Could you check a few things on this model? Use its own coordinates, in mm. A direction names the side the tool comes from. Round coordinates to 2 decimals unless told otherwise and drop trailing zeros. Loops run counter-clockwise (first coordinate to the right, second up) from the corner with the lowest first, then second, coordinate; pieces in that order, holes last. Notation, with made-up numbers: (86, 10) -> (100, 10) arc R23 ccw to (100, 20) -> close; hole circle Ø11 at (-4, 70). An arc over 180 degrees is marked (long way). Write each question's results on one line, items separated by ' | '. Start each with the question number.
1) Imagine slicing it at B-B, the plane x = -4. List the corners of the cut face in (y, z) for me, plus the area to 3 significant figures.
2) For P1, Ø2, axis at x = -17, y = 1, coming from the +Z side; P2, Ø3, axis at x = 12, y = 2.5, coming from the -Z side; P3, Ø0.9, axis at x = -1, z = 1.5, coming from the +Y side, each with a flat end and sliding along its axis, tell me the tip position at first contact or that it passes through.
3) If I drill on probe 1 along X at (y, z) = (0.8, 0); probe 2 along X at (y, z) = (0.5, 9.5); probe 3 along X at (y, z) = (1.5, 0), over which ranges is the centre line in solid material (lowest first)?
4) We'd pull the mould along Z, two halves only. Please class faces 3 (the cylindrical face through (0.07, 0.99, 10.6)), 4 (the flat face through (0.14, 3.521, -12.246)), 5 (the cylindrical face through (-22.497, 0.986, -0.275)): pulls with the +Z half, pulls with the -Z half, needs draft (parallel to the pull), parting line crosses it, or undercut.
5) Imagine slicing it at A-A, the plane z = 0. List the corners of the cut face in (x, y) for me, plus the area to 3 significant figures.
6) Which directions (+Z, -Z, +X, -X, +Y, -Y) give clear straight access to the entire face, cutting with the end or side of a thin tool? Please do faces 1 (the cylindrical face through (-19.27, 1.01, 1.22)), 2 (the flat face through (1, 2, -7)).
from build123d import *
from OCP.BRepFilletAPI import BRepFilletAPI_MakeChamfer

# Parameters (mm, degrees)
BOSS_EXTRUDE1_DEPTH = 2
SKETCH2_R           = 9.349999999999996
CUT_EXTRUDE1_DEPTH  = 26.81666128685116
BOSS_EXTRUDE2_DEPTH = 3
CHAMFER1_SIZE       = 3
CHAMFER1_SIZE2      = 0.5
SKETCH4_W           = 15.000000000000002
SKETCH4_H           = 12
CUT_EXTRUDE2_DEPTH  = 1
CHAMFER2_SIZE       = 1
CHAMFER2_SIZE_2     = 2
SKETCH5_R           = 1.6000000000000005
SKETCH5_R_2         = 0.75
SKETCH5_R_3         = 0.7500000000000004
CUT_EXTRUDE3_DEPTH  = 27.22022120425378


with BuildPart() as part:
    # Sketch1 → Boss-Extrude1 (new body)
    with BuildSketch(Plane(origin=(0, 0, 0), x_dir=(1, 0, 0), z_dir=(0, 1, 0))):
        with BuildLine():
            Line((-22.5, 0), (-10, 0))
            Line((-10, 0), (1.421e-14, 0))
            Line((1.351e-14, 0), (-3.6e-16, 12.499999999999996))
            Line((0, 12.499999999999996), (-9.999999999999998, 12.499999999999996))
            ThreePointArc((-10.000000000000007, 12.499999999999996), (-18.83883476483184, 8.83883476483184), (-22.499999999999993, 7.9e-16))
        make_face()
        with BuildLine():
            Line((1.421e-14, 0), (-10, 0))
            Line((-10, 0), (-22.5, 0))
            ThreePointArc((-22.499999999999993, 7.9e-16), (-18.83883476483183, -8.83883476483185), (-9.999999999999972, -12.499999999999993))
            Line((-9.999999999999973, -12.499999999999996), (2.665e-14, -12.499999999999996))
            Line((2.739e-14, -12.499999999999996), (1.351e-14, 0))
        make_face()
        with BuildLine():
            Line((10, 0), (1.421e-14, 0))
            Line((1.351e-14, 0), (2.739e-14, -12.499999999999996))
            Line((2.665e-14, -12.499999999999996), (10.000000000000012, -12.499999999999996))
            ThreePointArc((10.000000000000012, -12.499999999999995), (18.838834764831844, -8.838834764831835), (22.499999999999993, 1.01e-15))
            Line((22.5, 0), (10, 0))
        make_face()
        with BuildLine():
            Line((-3.6e-16, 12.499999999999996), (1.351e-14, 0))
            Line((1.421e-14, 0), (10, 0))
            Line((10, 0), (22.5, 0))
            ThreePointArc((22.499999999999993, 1.01e-15), (18.83883476483184, 8.83883476483184), (10, 12.499999999999995))
            Line((9.999999999999998, 12.499999999999996), (0, 12.499999999999996))
        make_face()
    extrude(amount=BOSS_EXTRUDE1_DEPTH)

    # Sketch2 → Cut-Extrude1 (cut, through all)
    with BuildSketch(Plane(origin=(0, 2, 0), x_dir=(1, 0, 0), z_dir=(0, 1, 0))):
        with Locations(Location((10, 0, 0), (0, 0, 270))):
            Circle(SKETCH2_R)
        with Locations(Location((-10, 0, 0), (0, 0, 90))):
            Circle(SKETCH2_R)
    extrude(amount=-CUT_EXTRUDE1_DEPTH, mode=Mode.SUBTRACT)

    # Sketch3 → Boss-Extrude2 (add)
    with BuildSketch(Plane(origin=(0, 2, 0), x_dir=(1, 0, 0), z_dir=(0, 1, 0))):
        with BuildLine():
            Line((-9.99999999999998, -12.499999999999996), (10.000000000000009, -12.499999999999996))
            ThreePointArc((10.000000000000009, -12.499999999999996), (22.499999999999996, 2.78e-15), (10, 12.499999999999996))
            Line((10, 12.499999999999996), (-9.999999999999998, 12.499999999999996))
            ThreePointArc((-9.999999999999998, 12.499999999999996), (-22.499999999999996, -9.57e-15), (-9.99999999999998, -12.499999999999996))
        make_face()
        with BuildLine():
            Line((9.999999999999998, 11.499999999999996), (-9.999999999999998, 11.499999999999996))
            ThreePointArc((-9.999999999999998, 11.499999999999996), (-21.499999999999996, -8.81e-15), (-9.99999999999998, -11.499999999999996))
            Line((-9.99999999999998, -11.499999999999996), (10.000000000000012, -11.499999999999996))
            ThreePointArc((10.000000000000012, -11.499999999999996), (21.499999999999996, 7.66e-15), (9.999999999999998, 11.499999999999996))
        make_face(mode=Mode.SUBTRACT)
    extrude(amount=BOSS_EXTRUDE2_DEPTH)

    # Chamfer1: one chamfer whose edges measure the first distance from different faces: ONE call of the kernel's chamfer builder (chamfer() names one face for all edges)
    chamfer1_edges_1 = [part.edges().sort_by_distance(p)[0] for p in [
        (22.5, 5, -1.79e-15),
    ]]
    chamfer1_side_1 = [part.faces().sort_by_distance(p)[0] for p in [
        (22.499999999999993, 2.5, -1.478e-14),
    ]]
    chamfer1_edges_2 = [part.edges().sort_by_distance(p)[0] for p in [
        (0, 5, -12.499999999999996),
    ]]
    chamfer1_side_2 = [part.faces().sort_by_distance(p)[0] for p in [
        (-4.6e-16, 2.5, -12.499999999999996),
    ]]
    chamfer1_edges_3 = [part.edges().sort_by_distance(p)[0] for p in [
        (-22.499999999999993, 5, 1.178e-14),
    ]]
    chamfer1_side_3 = [part.faces().sort_by_distance(p)[0] for p in [
        (-22.499999999999993, 2.5, 1.611e-14),
    ]]
    chamfer1_edges_4 = [part.edges().sort_by_distance(p)[0] for p in [
        (1.421e-14, 5, 12.499999999999996),
    ]]
    chamfer1_side_4 = [part.faces().sort_by_distance(p)[0] for p in [
        (1.744e-14, 2.5, 12.499999999999996),
    ]]
    chamfer1 = BRepFilletAPI_MakeChamfer(part.part.solid().wrapped)
    for e in chamfer1_edges_1:
        chamfer1.Add(CHAMFER1_SIZE, CHAMFER1_SIZE2, e.wrapped, chamfer1_side_1[0].wrapped)  # the first distance lies on this face
    for e in chamfer1_edges_2:
        chamfer1.Add(CHAMFER1_SIZE, CHAMFER1_SIZE2, e.wrapped, chamfer1_side_2[0].wrapped)  # the first distance lies on this face
    for e in chamfer1_edges_3:
        chamfer1.Add(CHAMFER1_SIZE, CHAMFER1_SIZE2, e.wrapped, chamfer1_side_3[0].wrapped)  # the first distance lies on this face
    for e in chamfer1_edges_4:
        chamfer1.Add(CHAMFER1_SIZE, CHAMFER1_SIZE2, e.wrapped, chamfer1_side_4[0].wrapped)  # the first distance lies on this face
    add(Compound.cast(chamfer1.Shape()), mode=Mode.REPLACE)

    # Sketch4 → Cut-Extrude2 (cut)
    with BuildSketch(Plane(origin=(0, 2, 0), x_dir=(1, 0, 0), z_dir=(0, 1, 0))):
        Rectangle(SKETCH4_W, SKETCH4_H)
    extrude(amount=-CUT_EXTRUDE2_DEPTH, mode=Mode.SUBTRACT)

    # Chamfer2
    chamfer2_edges_1 = [part.edges().sort_by_distance(p)[0] for p in [
        (-8.9e-16, 1, 6),
    ]]
    chamfer2_side_1 = [part.faces().sort_by_distance(p)[0] for p in [
        (-8.9e-16, 1.02, 6),
    ]]
    chamfer2_edges_2 = [part.edges().sort_by_distance(p)[0] for p in [
        (8.9e-16, 1, -6),
    ]]
    chamfer2_side_2 = [part.faces().sort_by_distance(p)[0] for p in [
        (8.9e-16, 1, -5.98),
    ]]
    chamfer2 = BRepFilletAPI_MakeChamfer(part.part.solid().wrapped)
    for e in chamfer2_edges_1:
        chamfer2.Add(CHAMFER2_SIZE - 0.0001, CHAMFER2_SIZE_2 - 0.0001, e.wrapped, chamfer2_side_1[0].wrapped)
    for e in chamfer2_edges_2:
        chamfer2.Add(CHAMFER2_SIZE_2 - 0.0001, CHAMFER2_SIZE - 0.0001, e.wrapped, chamfer2_side_2[0].wrapped)
    add(Compound.cast(chamfer2.Shape()), mode=Mode.REPLACE)  # a hair under: the kernel refuses the full size

    # Sketch5 → Cut-Extrude3 (cut, through all)
    with BuildSketch(Plane.XZ):
        with Locations(Location((0, 8.999999999999998, 0), (0, 0, 270))):
            Circle(SKETCH5_R)
        with Locations(Location((-4.000000000000002, 9.499999999999998, 0), (0, 0, 270))):
            Circle(SKETCH5_R_2)
        with Locations(Location((3.9999999999999982, 9.499999999999998, 0), (0, 0, 270))):
            Circle(SKETCH5_R_3)
    extrude(amount=-CUT_EXTRUDE3_DEPTH, mode=Mode.SUBTRACT)


solid = part.part
Checked values:
1) outline: (0, -12.5) -> (2, -12.5) -> (5, -12) -> (5, -11.5) -> (2, -11.5) -> (2, -7.17) -> (0, -7.17) -> close; (0, 7.17) -> (2, 7.17) -> (2, 8.75) -> (0, 8.75) -> close; (0, 10.25) -> (2, 10.25) -> (2, 11.5) -> (5, 11.5) -> (5, 12) -> (2, 12.5) -> (0, 12.5) -> close | area: 22.8 mm^2
2) P1: z = 10.97 | P2: z = -12.49 | P3: y = 1
3) probe 1: -22.5 to -19.35, -0.65 to 0.65, 19.35 to 22.5 | probe 2: -18.12 to -4.75, -3.25 to -1.52, 1.52 to 3.25, 4.75 to 18.12 | probe 3: -22.5 to -19.35, 19.35 to 22.5
4) face 3: undercut | face 4: pulls with the -Z half | face 5: parting line crosses it
5) outline: (-22.5, 0) -> (-19.35, 0) -> (-19.35, 2) -> (-21.5, 2) -> (-21.5, 5) -> (-22, 5) -> (-22.5, 2) -> close; (-0.65, 0) -> (0.65, 0) -> (0.65, 1) -> (-0.65, 1) -> close; (19.35, 0) -> (22.5, 0) -> (22.5, 2) -> (22, 5) -> (21.5, 5) -> (21.5, 2) -> (19.35, 2) -> close | area: 18.4 mm^2
6) face 1: +Y, -Y | face 2: +Y
